Study the drawing (mm; zero at the part's minimum x, y, z) and answer. A direction names the side the tool comes from. Give positions to 0.01 mm unless a question says otherwise; leave off trailing zeros. Order: outer loops, then holes, each group sorted by start corner. A loop starts at its lowest first (then second) coordinate and runs counter-clockwise, first axis right, second up. Notation, with made-up numbers: (39.25, 62) - (70.25, 62) arc R18 ccw to (70.25, 70) - close; hole circle Ø11 at (-32.75, 77.25). An arc over 180 degrees is marked (long way). Return JSON: item names as keys, results as strings.
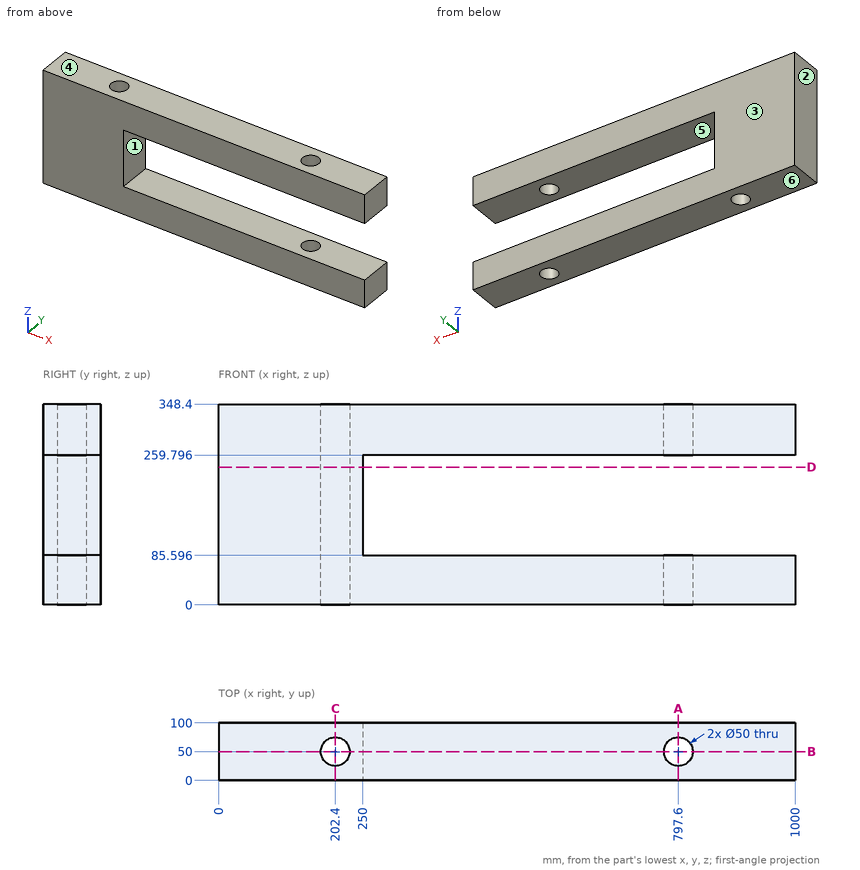
Q1. A cutting plane is placed at B-B (y = 50). Write down the section's boundary in (x, z).
Values:
{"outline": "(0, 0) - (177.4, 0) - (177.4, 348.4) - (0, 348.4) - close; (227.4, 0) - (772.6, 0) - (772.6, 85.6) - (250, 85.6) - (250, 259.8) - (772.6, 259.8) - (772.6, 348.4) - (227.4, 348.4) - close; (822.6, 0) - (1000, 0) - (1000, 85.6) - (822.6, 85.6) - close; (822.6, 259.8) - (1000, 259.8) - (1000, 348.4) - (822.6, 348.4) - close"}
Q2. Determine the mould class of the marked faces 3, 4, 5 and 6 for opening direction Z: released by +Z, released by -Z, zero draft, split by the parting line, or undercut.
Values:
{"face 3": "zero draft", "face 4": "released by +Z", "face 5": "undercut", "face 6": "released by -Z"}
Q3. For the marked faces 1 and 2, determine the directions among +Z, -Z, +X, -X, +Y, -Y from which every point of the face is accessible in a straight line to the end or side of a thin tool.
Values:
{"face 1": "+X, +Y, -Y", "face 2": "+Z, -Z, -X, +Y, -Y"}
Q4. Given pin 1 (5 mm diameter, centred on y = 23, z = 249.5, fed in from +X), flat-ended and moving along its own axis, determine where the tip first touches the part or whether it passes through.
Values:
{"pin 1": "stops at x = 250"}
Q5. Consider L1, parallel to Z at x = 385, y = 46; L2, parallel to Y at x = 797, z = 314; L3, parallel to X at y = 56, z = 281. Determine where each line is inside the solid, lowest interval first.
Values:
{"L1": "z = 0 to 85.6, 259.8 to 348.4", "L2": "y = 0 to 25.01, 74.99 to 100", "L3": "x = 0 to 178.13, 226.67 to 773.33, 821.87 to 1000"}
Q6. A cutting plane is placed at D-D (z = 239). Write down the section's boundary in (x, y), and give its area (3 significant figures).
Values:
{"outline": "(0, 0) - (250, 0) - (250, 100) - (0, 100) - close; hole circle Ø50 at (202.4, 50)", "area": "23,000 mm²"}
Q7. A cutting plane is placed at A-A (x = 797.6). Write down the section's boundary in (y, z), and give its area (3 significant figures).
Values:
{"outline": "(0, 0) - (25, 0) - (25, 85.6) - (0, 85.6) - close; (0, 259.8) - (25, 259.8) - (25, 348.4) - (0, 348.4) - close; (75, 0) - (100, 0) - (100, 85.6) - (75, 85.6) - close; (75, 259.8) - (100, 259.8) - (100, 348.4) - (75, 348.4) - close", "area": "8,710 mm²"}
Q8. A cutting plane is placed at C-C (x = 202.4). Write down the section's boundary in (y, z), and give its area (3 significant figures).
Values:
{"outline": "(0, 0) - (25, 0) - (25, 348.4) - (0, 348.4) - close; (75, 0) - (100, 0) - (100, 348.4) - (75, 348.4) - close", "area": "17,400 mm²"}
